from build123d import *

# Parameters (mm, degrees)
SKETCH1_R           = 30
BOSS_EXTRUDE1_DEPTH = 5
SKETCH2_W           = 60
SKETCH2_H           = 40
BOSS_EXTRUDE2_DEPTH = 5
SKETCH3_R           = 1.45
CUT_EXTRUDE1_DEPTH  = 5
SKETCH4_R           = 1.45
BOSS_EXTRUDE3_DEPTH = 4
SKETCH5_W           = 22
SKETCH5_H           = 11.5
BOSS_EXTRUDE4_DEPTH = 108.5


with BuildPart() as part:
    # Sketch1 → Boss-Extrude1 (new body)
    with BuildSketch(Plane.XY.offset(384.5)):
        with Locations((300, 300)):
            Circle(SKETCH1_R)
    extrude(amount=BOSS_EXTRUDE1_DEPTH)

    # Sketch2 → Boss-Extrude2 (add)
    with BuildSketch(Plane.XY.offset(384.5)):
        with Locations((300, 320)):
            Rectangle(SKETCH2_W, SKETCH2_H)
    extrude(amount=BOSS_EXTRUDE2_DEPTH)

    # Sketch3 → Cut-Extrude1 (cut)
    with BuildSketch(Plane.XY.offset(384.5)):
        with Locations((286.774831823, 318.202882373)):
            Circle(SKETCH3_R)
        with Locations((278.601228383, 293.047117627)):
            Circle(SKETCH3_R)
        with Locations((300, 277.5)):
            Circle(SKETCH3_R)
        with Locations((321.398771617, 293.047117627)):
            Circle(SKETCH3_R)
        with Locations((313.225168177, 318.202882373)):
            Circle(SKETCH3_R)
        with BuildLine():
            Line((292.928932188, 292.928932188), (300, 285.857864376))
            Line((300, 285.857864376), (307.071067812, 292.928932188))
            ThreePointArc((307.071067812, 292.928932188), (300, 310), (292.928932188, 292.928932188))
        make_face()
    extrude(amount=CUT_EXTRUDE1_DEPTH, mode=Mode.SUBTRACT)



with BuildPart() as body_2:
    # Sketch4 → Boss-Extrude3 (new body)
    with BuildSketch(Plane.XY.offset(276)):
        Polygon((289, 340), (311, 340), (311, 334), (330, 315), (330, 270), (270, 270), (270, 315), (289, 334), align=None)
        with Locations((286.774831823, 318.202882373)):
            Circle(SKETCH4_R, mode=Mode.SUBTRACT)
        with Locations((278.601228383, 293.047117627)):
            Circle(SKETCH4_R, mode=Mode.SUBTRACT)
        with Locations((300, 277.5)):
            Circle(SKETCH4_R, mode=Mode.SUBTRACT)
        with Locations((321.398771617, 293.047117627)):
            Circle(SKETCH4_R, mode=Mode.SUBTRACT)
        with Locations((313.225168177, 318.202882373)):
            Circle(SKETCH4_R, mode=Mode.SUBTRACT)
        with BuildLine():
            Line((292.928932188, 292.928932188), (300, 285.857864376))
            Line((300, 285.857864376), (307.071067812, 292.928932188))
            ThreePointArc((307.071067812, 292.928932188), (300, 310), (292.928932188, 292.928932188))
        make_face(mode=Mode.SUBTRACT)
    extrude(amount=BOSS_EXTRUDE3_DEPTH)


with BuildPart() as part_1:
    add(part.part)

    add(body_2.part)  # Boss-Extrude4 merges body 2
    # Sketch5 → Boss-Extrude4 (add)
    with BuildSketch(Plane.XY.offset(276)):
        with Locations((300, 334.25)):
            Rectangle(SKETCH5_W, SKETCH5_H)
    extrude(amount=BOSS_EXTRUDE4_DEPTH)


solid = part_1.part
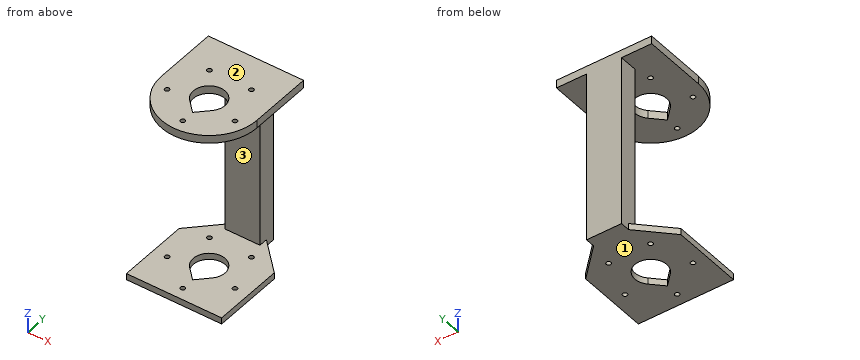
Check sheet for the modelled part. Datum: model origin and axes. Units: mm. Face numbers are marked on the shaded views. Round coordinates to 2 decimals unless told otherwise and drop trailing zeros. Order: outer loops, then holes, each group sorted by start corner. A loop starts at its lowest first (then second) coordinate and runs counter-clockwise, first axis right, second up.
Q1. Cross-section at B-B, the plane y = 304. Enter the section's corners in (x, z).
Filled sheet:
outline: (270, 276) - (290.83, 276) - (290.83, 280) - (270, 280) - close; (270, 384.5) - (290.83, 384.5) - (290.83, 389.5) - (270, 389.5) - close; (309.17, 276) - (330, 276) - (330, 280) - (309.17, 280) - close; (309.17, 384.5) - (330, 384.5) - (330, 389.5) - (309.17, 389.5) - close
Q2. Cross-section at A-A, the plane y = 324. Enter the section's corners in (x, z).
Filled sheet:
outline: (270, 384.5) - (330, 384.5) - (330, 389.5) - (270, 389.5) - close; (279, 276) - (321, 276) - (321, 280) - (279, 280) - close
Q3. Cross-section at C-C, the plane x = 283. Enter the section's corners in (y, z), plus the area to 3 significant figures.
Filled sheet:
outline: (270, 276) - (328, 276) - (328, 280) - (270, 280) - close; (275.28, 384.5) - (340, 384.5) - (340, 389.5) - (275.28, 389.5) - close
area: 556 mm2
Q4. Depth check by flat-ended pin: P1, Ø8, axis at x = 317, z = 369.5, coming from the +Y side; P2, Ø11, axis at x = 298, z = 316, coming from the -Y side; P3, Ø6, axis at y = 337, z = 317.5, coming from the -X side; P4, Ø3.5, axis at y = 335.5, z = 347.5, coming from the +X side. Enter the tip coordinate at first touch or a pass-through.
Filled sheet:
P1: passes through
P2: stops at y = 328.5
P3: stops at x = 289
P4: stops at x = 311
Q5. Scan lines: L1, parallel to Y at x = 300, z = 278.5; L2, parallel to Z at x = 311, y = 283; L3, parallel to Y at x = 291, z = 333.5. Record each from-to range of solid material in increasing order.
Filled sheet:
L1: y = 270 to 276.05, 278.95 to 285.86, 310 to 340
L2: z = 276 to 280, 384.5 to 389.5
L3: y = 328.5 to 340
Q6. Draft check along Z on the marked faces 1, 2 and 3. Enter one of: pulls with the +Z half, pulls with the -Z half, needs draft (parallel to the pull), parting line crosses it, or undercut.
Filled sheet:
face 1: pulls with the -Z half
face 2: pulls with the +Z half
face 3: undercut
Q7. Cross-section at D-D, the plane z = 364.5. Enter the section's corners in (x, y).
Filled sheet:
outline: (289, 328.5) - (311, 328.5) - (311, 340) - (289, 340) - close
